Could you check a few things on this model? Use its own coordinates, in mm. Face numbers are marked on the shaded views. A direction names the side the tool comes from. Round coordinates to 2 decimals unless told otherwise and drop trailing zeros. Loops run counter-clockwise (first coordinate to the right, second up) from the corner with the lowest first, then second, coordinate; pieces in that order, holes last. Notation, with made-up numbers: (-25, 3.25) -> (-2, 3.25) arc R26 cw to (-2, 42.25) -> close; hole circle Ø8 at (75.5, 35). An arc over 180 degrees is marked (long way). Put each result on its own line as item: value. Start each with the question number.
1. Imagine slicing it at B-B, the plane y = 20. Please give me the cut outline in (x, z) (3 decimals), and give its area (3 significant figures).
2. I'm going to push flat-ended pins straight in: P1, Ø3, axis at x = 3.5, y = 16.5, coming from the +Z side; P2, Ø4, axis at x = -23, z = 5, coming from the -Y side; P3, Ø4, axis at y = -9, z = 5, coming from the -X side. Where does each tip first touch, or does it pass through?
3. I need wall thicknesses on line 1 (Z direction, x = -7, y = -20); line 2 (Y direction, x = 19, z = 2.5); line 3 (X direction, y = 8.5, z = 2.5). Which ranges of each line are inside material? Lowest first, please. Write a range as [from, to].
4. Imagine slicing it at C-C, the plane z = 3.25. Please give me the cut outline in (x, y), and give its area (3 significant figures).
5. Which directions (+Z, -Z, +X, -X, +Y, -Y) give clear straight access to the entire face, cutting with the end or side of a thin tool? Please do the marked faces 1 and 2.
6. Imagine slicing it at A-A, the plane x = 0. Please give me the cut outline in (y, z) (3 decimals), and give its area (3 significant figures).
7. Imagine slicing it at D-D, the plane z = 6.5. Please give me the cut outline in (x, y) (3 decimals), and give its area (3 significant figures).
```python
from build123d import *

# Parameters (mm, degrees)
SKETCH1_R           = 30
BOSS_EXTRUDE1_DEPTH = 5
SKETCH2_R           = 2.875
BOSS_EXTRUDE2_DEPTH = 5
SKETCH3_R           = 2.390739662
CUT_EXTRUDE1_DEPTH  = 10


with BuildPart() as part:
    # Sketch1 → Boss-Extrude1 (new body)
    with BuildSketch(Plane.XY):
        Circle(SKETCH1_R)
    extrude(amount=BOSS_EXTRUDE1_DEPTH)

    # Sketch2 → Boss-Extrude2 (add)
    with BuildSketch(Plane.XY.offset(5)):
        with Locations((0, 20)):
            Circle(SKETCH2_R)
    extrude(amount=BOSS_EXTRUDE2_DEPTH)

    # Sketch3 → Cut-Extrude1 (cut)
    with BuildSketch(Plane.XY.offset(5)):
        with Locations((-16.548801548, -13.666947255)):
            Circle(SKETCH3_R)
    extrude(amount=-CUT_EXTRUDE1_DEPTH, mode=Mode.SUBTRACT)


solid = part.part
```
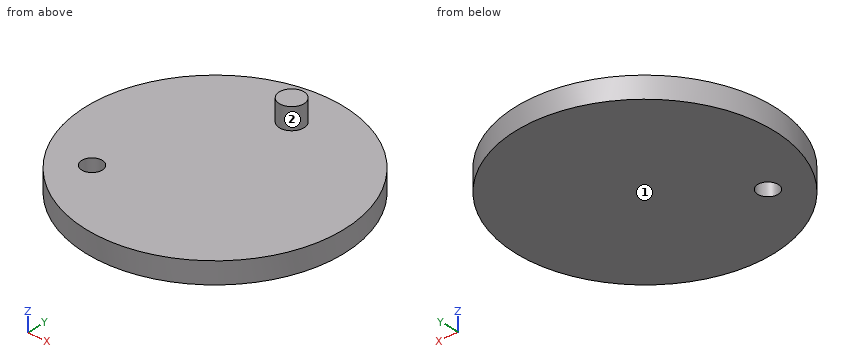
Entries:
1. outline: (-22.361, 0) -> (22.361, 0) -> (22.361, 5) -> (2.875, 5) -> (2.875, 10) -> (-2.875, 10) -> (-2.875, 5) -> (-22.361, 5) -> close
1. area: 252 mm^2
2. P1: z = 5
2. P2: y = -21.42
2. P3: x = -29.17
3. line 1: [0, 5]
3. line 2: [-23.22, 23.22]
3. line 3: [-28.77, 28.77]
4. outline: circle Ø60 at (0, 0); hole circle Ø4.78 at (-16.55, -13.67)
4. area: 2,810 mm^2
5. face 1: -Z, +X, -X, +Y, -Y
5. face 2: +Z
6. outline: (-30, 0) -> (30, 0) -> (30, 5) -> (22.875, 5) -> (22.875, 10) -> (17.125, 10) -> (17.125, 5) -> (-30, 5) -> close
6. area: 329 mm^2
7. outline: circle Ø5.75 at (0, 20)
7. area: 26.0 mm^2
